Verification items for the finished model (mm, model axes). A direction names the side the tool comes from. Coordinates: 2 decimals unless noted, no trailing zeros. Write each question's results on one line, items separated by ' | '. Start each with the question number.
(1) Thickness scan on probe 1 along X at (y, z) = (-15.5, 12.7); probe 2 along X at (y, z) = (5.25, 12.7); probe 3 along Z at (x, y) = (0, -15.8). Record the ranges inside material, lowest first. Write a range as [from, to].
(2) Set-up check for faces 1 (the cylindrical face through (-1.393, 0.027, -63.325)), 2 (the cylindrical face through (-0.168, 6.781, -53.344)), 3 (the flat face through (50.8, -3, 9)), 4 (the flat face through (63.5, -3, 9)): record each of +Z, -Z, +X, -X, +Y, -Y from which the full face is reachable in a straight line by a thin tool's end or side.
(3) Draft check along Z on faces 5 (the flat face through (-57, 3.65, 10)), 6 (the flat face through (-63.5, -8, 9)), 7 (the flat face through (2, 3.65, -59)), 8 (the conical face through (-1.041, -4.242, -47.341)). Enter one of: +Z half, -Z half, draft (parallel to the pull), parting line (faces both ways), or undercut.
(4) Go/stop test with flat-tipped pins: pin 1 (1.8 mm diameter, centred on x = -49.5, y = -6, fed in from +Z); pin 2 (2.5 mm diameter, centred on x = -1.5, z = -58.5, fed in from +Y); pin 3 (3 mm diameter, centred on y = -0.5, z = 6.5, fed in from +X). Record where each tip stops, or that it passes through.
(5) Cross-section at A-A on z = 12.7. Give the number of separate pieces and of enclosed holes in the cut face, and give its area (3 significant figures).
```python
from build123d import *

# Parameters (mm, degrees)
REVOLVE1_ANGLE          = 180
BOSS_EXTRUDE1_DEPTH     = 5.08
BOSS_EXTRUDE2_OUTLINE_W = 12.7
BOSS_EXTRUDE2_OUTLINE_H = 25.08
BOSS_EXTRUDE2_DEPTH     = 19.05
CUT_EXTRUDE2_DEPTH      = 99.22042252
CUT_EXTRUDE2_DEPTH_BACK = 99.22042252
SKETCH5_R               = 2.2225
CUT_EXTRUDE3_DEPTH      = 99.22042252
CUT_EXTRUDE3_DEPTH_BACK = 6.35
SKETCH7_R               = 3.81
BOSS_EXTRUDE3_START     = 1.143
SKETCH5_8_R             = 2.2225
BOSS_EXTRUDE3_DEPTH     = 1.143


# Read off the part's stored shape, not the designer's step: Boss-Extrude2
with BuildPart() as part:
    # Sketch1 → Revolve1 (revolve)
    with BuildSketch(Plane.XY):
        Polygon((-67.15, 10), (-47.15, 10), (-47.15, 4.445), (-48.42, 3.175), (-49.69, 3.175), (-50.96, 1.905), (-50.96, -1.905), (-49.69, -3.175), (-48.42, -3.175), (-47.15, -4.445), (-47.15, -10), (-67.15, -10), (-67.15, -4.445), (-65.88, -3.175), (-64.61, -3.175), (-63.34, -1.905), (-63.34, 1.905), (-64.61, 3.175), (-65.88, 3.175), (-67.15, 4.445), align=None)
    revolve(axis=Axis((0, 0, 0), (0, -1, 0)), revolution_arc=REVOLVE1_ANGLE)

    # Sketch3 → Boss-Extrude1 (add)
    with BuildSketch(Plane.XZ.offset(10)):
        with BuildLine():
            Line((-47.15, 0), (-67.15, 0))
            ThreePointArc((-67.15, 0), (0, -67.15), (67.15, 0))
            Line((67.15, 0), (47.15, 0))
            ThreePointArc((47.15, 0), (0, -47.15), (-47.15, 0))
        make_face()
    extrude(amount=BOSS_EXTRUDE1_DEPTH)

    # Boss-Extrude2 outline → Boss-Extrude2 (add)
    with BuildSketch(Plane.XY):
        Polygon((-50.8, 10), (-63.5, 10), (-63.5, 2.065), (-63.34, 1.905), (-63.34, -1.905), (-63.5, -2.065), (-63.5, -15.08), (-50.8, -15.08), (-50.8, -2.065), (-50.96, -1.905), (-50.96, 1.905), (-50.8, 2.065), align=None)
        with Locations((57.15, -2.54)):
            Rectangle(BOSS_EXTRUDE2_OUTLINE_W, BOSS_EXTRUDE2_OUTLINE_H)
    extrude(amount=BOSS_EXTRUDE2_DEPTH)

    # Sketch5 → Cut-Extrude2 (cut, two sides: drawn at the far end of the back side and taken through both)
    with BuildSketch(Plane.XZ.offset(15.08).offset(-CUT_EXTRUDE2_DEPTH_BACK)):
        with BuildLine():
            ThreePointArc((-54.9275, 12.7), (-55.578455179, 14.271544821), (-57.15, 14.9225))
            Line((-57.15, 14.9225), (-57.15, 10.4775))
            ThreePointArc((-57.15, 10.4775), (-55.578455179, 11.128455179), (-54.9275, 12.7))
        make_face()
        with BuildLine():
            Line((-57.15, 10.4775), (-57.15, 14.9225))
            ThreePointArc((-57.15, 14.9225), (-59.3725, 12.7), (-57.15, 10.4775))
        make_face()
        with Locations(Location((0, -57.15, 0), (0, 0, 270))):
            Circle(SKETCH5_R)
        with Locations(Location((57.15, 12.7, 0), (0, 0, 270))):
            Circle(SKETCH5_R)
    extrude(amount=CUT_EXTRUDE2_DEPTH + CUT_EXTRUDE2_DEPTH_BACK, mode=Mode.SUBTRACT)

    # Sketch7 → Cut-Extrude3 (cut, two sides: drawn at the far end of the back side and taken through both)
    with BuildSketch(Plane(origin=(0, 10, 0), x_dir=(1, 0, 0), z_dir=(0, 1, 0)).offset(-CUT_EXTRUDE3_DEPTH_BACK)):
        with Locations(Location((0, 57.15, 0), (0, 0, 90))):
            Circle(SKETCH7_R)
        with Locations(Location((-57.15, -12.7, 0), (0, 0, 90))):
            Circle(SKETCH7_R)
        with Locations(Location((57.15, -12.7, 0), (0, 0, 90))):
            Circle(SKETCH7_R)
    extrude(amount=CUT_EXTRUDE3_DEPTH + CUT_EXTRUDE3_DEPTH_BACK, mode=Mode.SUBTRACT)

    # Sketch5<8> → Boss-Extrude3 (add)
    # profile 1 of 3: a face of its own
    with BuildSketch(Plane.XZ.offset(15.08).offset(BOSS_EXTRUDE3_START)):
        Polygon((-57.15, 16.54948292), (-60.48375, 14.62474146), (-60.48375, 10.77525854), (-57.15, 8.85051708), (-53.81625, 10.77525854), (-53.81625, 14.62474146), align=None)
        with Locations(Location((-57.15, 12.7, 0), (0, 0, 270))):
            Circle(SKETCH5_8_R, mode=Mode.SUBTRACT)
    # profile 2 of 3: a face of its own
    with BuildSketch(Plane.XZ.offset(15.08).offset(BOSS_EXTRUDE3_START)):
        Polygon((0, -60.99948292), (3.33375, -59.07474146), (3.33375, -55.22525854), (0, -53.30051708), (-3.33375, -55.22525854), (-3.33375, -59.07474146), align=None)
        with Locations(Location((0, -57.15, 0), (0, 0, 270))):
            Circle(SKETCH5_8_R, mode=Mode.SUBTRACT)
    # profile 3 of 3: a face of its own
    with BuildSketch(Plane.XZ.offset(15.08).offset(BOSS_EXTRUDE3_START)):
        Polygon((53.81625, 14.62474146), (57.15, 16.54948292), (60.48375, 14.62474146), (60.48375, 10.77525854), (57.15, 8.85051708), (53.81625, 10.77525854), align=None)
        with Locations(Location((57.15, 12.7, 0), (0, 0, 270))):
            Circle(SKETCH5_8_R, mode=Mode.SUBTRACT)
    extrude(amount=-BOSS_EXTRUDE3_DEPTH)


solid = part.part
```
Results are:
1) probe 1: x = [-60.48, -59.37], [-54.93, -53.82], [53.82, 54.93], [59.37, 60.48] | probe 2: x = [-63.5, -60.96], [-53.34, -50.8], [50.8, 53.34], [60.96, 63.5] | probe 3: z = [-61, -59.37], [-54.93, -53.3]
2) face 1: -Z | face 2: +Y | face 3: +Z, +Y, -Y | face 4: +Z, +X, +Y, -Y
3) face 5: undercut | face 6: draft | face 7: undercut | face 8: +Z half
4) pin 1: stops at z = 0 | pin 2: stops at y = 3.65 | pin 3: stops at x = 63.5
5) separate pieces: 4 | enclosed holes: 0 | area: 378 mm2
